from build123d import *

# Parameters (mm, degrees)
EXTRUDE_2_DEPTH     = 330
SKETCH_2_W          = 66
SKETCH_2_H          = 220
SKETCH_2_W_2        = 145
SKETCH_2_H_2        = 100
CUT_EXTRUDE_1_DEPTH = 10
SKETCH_5_W          = 82
SKETCH_5_H          = 220
CUT_EXTRUDE_3_DEPTH = 10
SKETCH_9_W          = 65
SKETCH_9_H          = 220
CUT_EXTRUDE_5_DEPTH = 10


with BuildPart() as part:
    # Эскиз1 → Вытянуть-Тонкостенный2 (new body)
    with BuildSketch(Plane(origin=(0, 0, 0), x_dir=(1, 0, 0), z_dir=(0, 1, 0))):
        Polygon((-34.007352544, 521), (-351, 521), (-351, -1), (1, -1), (1, 66), (-139.537591907, 66), (-207.007352544, 145.367607311), (-207.007352544, 160), (-237.007352544, 160), (-237.007352544, 248), (-204.007352544, 248), (-204.007352544, 265), (-34.007352544, 265), align=None)
        Polygon((-35.007352544, 520), (-350, 520), (-350, 0), (0, 0), (0, 65), (-140, 65), (-208.007352544, 145), (-208.007352544, 159), (-238.007352544, 159), (-238.007352544, 249), (-205.007352544, 249), (-205.007352544, 266), (-35.007352544, 266), align=None, mode=Mode.SUBTRACT)
    extrude(amount=EXTRUDE_2_DEPTH)

    # Эскиз2 → Вырез-Вытянуть1 (cut)
    with BuildSketch(Plane(origin=(0, 0, -521), x_dir=(-1, 0, 0), z_dir=(0, 0, -1))):
        with Locations((249, 120)):
            Rectangle(SKETCH_2_W, SKETCH_2_H)
        with Locations((113.5, 150)):
            Rectangle(SKETCH_2_W_2, SKETCH_2_H_2)
    extrude(amount=-CUT_EXTRUDE_1_DEPTH, mode=Mode.SUBTRACT)

    # Эскиз5 → Вырез-Вытянуть3 (cut)
    with BuildSketch(Plane.ZY.offset(351)):
        with Locations((-83, 120)):
            Rectangle(SKETCH_5_W, SKETCH_5_H)
    extrude(amount=-CUT_EXTRUDE_3_DEPTH, mode=Mode.SUBTRACT)

    # Эскиз9 → Вырез-Вытянуть5 (cut)
    with BuildSketch(Plane(origin=(-49.193811045, 0, 41.819260634), x_dir=(0.6476890718445449, 0, 0.7619047619047621), z_dir=(-0.7619047619047621, 0, 0.6476890718445449))):
        with Locations((-202.700279582, 120)):
            Rectangle(SKETCH_9_W, SKETCH_9_H)
    extrude(amount=-CUT_EXTRUDE_5_DEPTH, mode=Mode.SUBTRACT)


solid = part.part
Here's how the part is built. I have some questions about the finished solid (model axes, mm). A direction names the side the tool comes from. Coordinates: 2 decimals unless noted, no trailing zeros. Loops run counter-clockwise (first coordinate to the right, second up) from the corner with the lowest first, then second, coordinate; pieces in that order, holes last.
1. Imagine slicing it at A-A, the plane z = -288. Please give me the cut outline in (x, y), and give its area (3 significant figures).
2. I need wall thicknesses on L1, parallel to Z at x = -222, y = 211; L2, parallel to Z at x = -61.5, y = 106.5; L3, parallel to Z at x = -52, y = 261.5. Which ranges of each line are inside material? Lowest first, please.
3. Imagine slicing it at D-D, the plane x = -252.5. Please give me the cut outline in (y, z).
4. For faces 1 (the flat face through (1, 163, -32)), 2 (the flat face through (-222, 163, -249)), 3 (the flat face through (-221, 163, -248)), which set-ups out of +Z, -Z, +X, -X, +Y, -Y let a thin tool reach every point of the face, with its end or its side?
5. Imagine slicing it at C-C, the plane y = 237. Please give me the cut outline in (x, z).
6. For P1, Ø1.5, axis at x = -252.5, y = 153, coming from the -Z side; P2, Ø7.5, axis at y = 135.5, z = -150, coming from the +X side; P3, Ø8.5, axis at y = 147.5, z = -253.5, coming from the +X side, each with a flat end and sliding along its axis, tell me the tip position at first contact or that it passes through.
7. Imagine slicing it at B-B, the plane x = -170.5. Please give me the cut outline in (y, z), and give its area (3 significant figures).
8. If we mould it in two halves opening along Z, with no side actions, what happens to faces 4 (the flat face through (-222, 163, -160)), 5 (the flat face through (-177, 163, 1)), 6 (the flat face through (-34.007, 163, -391))? For each: pulls with the +Z half, pulls with the -Z half, needs draft (parallel to the pull), parting line crosses it, or undercut.
Taken from the geometry:
1. outline: (-351, 0) - (-350, 0) - (-350, 330) - (-351, 330) - close; (-35.01, 0) - (-34.01, 0) - (-34.01, 330) - (-35.01, 330) - close
1. area: 660 mm2
2. L1: z = -249 to -248, -160 to -159, 0 to 1
2. L2: z = -266 to -265, -66 to -65, 0 to 1
2. L3: z = -521 to -520, -266 to -265, -66 to -65, 0 to 1
3. outline: (0, -521) - (10, -521) - (10, -520) - (0, -520) - close; (0, 0) - (330, 0) - (330, 1) - (0, 1) - close; (230, -521) - (330, -521) - (330, -520) - (230, -520) - close
4. face 1: +Z, -Z, +X, +Y, -Y
4. face 2: +Y, -Y
4. face 3: +X, +Y, -Y
5. outline: (-351, -521) - (-34.01, -521) - (-34.01, -265) - (-204.01, -265) - (-204.01, -248) - (-237.01, -248) - (-237.01, -160) - (-207.01, -160) - (-207.01, -145.37) - (-139.54, -66) - (1, -66) - (1, 1) - (-351, 1) - close; hole (-350, -520) - (-35.01, -520) - (-35.01, -266) - (-205.01, -266) - (-205.01, -249) - (-238.01, -249) - (-238.01, -159) - (-208.01, -159) - (-208.01, -145) - (-140, -65) - (0, -65) - (0, 0) - (-350, 0) - close
6. P1: stops at z = 0
6. P2: stops at x = -207.01
6. P3: stops at x = -204.01
7. outline: (0, -521) - (100, -521) - (100, -520) - (0, -520) - close; (0, -266) - (330, -266) - (330, -265) - (0, -265) - close; (0, -102.42) - (10, -102.42) - (10, -100.88) - (0, -100.88) - close; (0, 0) - (330, 0) - (330, 1) - (0, 1) - close; (200, -521) - (330, -521) - (330, -520) - (200, -520) - close; (230, -102.42) - (330, -102.42) - (330, -100.88) - (230, -100.88) - close
7. area: 1,060 mm2
8. face 4: undercut
8. face 5: pulls with the +Z half
8. face 6: needs draft
